For this review, take the finished solid that the model builds, in its own axes (mm). Give positions to 0.01 mm unless a question says otherwise; leave off trailing zeros. Write each loop counter-clockwise with the first axis right and the second up, starting at its lowest first coordinate (ties: lowest second). Pieces come first, ordered by that corner, then holes. Notation, with made-up numbers: M 15.25,-8 L 35.25,-8 A18 ccw 35.25,21 Z; hole C 65.25,74 d1. An arc over 180 degrees is marked long. One line per item, written item: value. Start each with the question number.
Item 1: Consider section B-B, the plane y = -89. Write out the cut boundary in (x, z), and give its area (3 significant figures).
Item 2: Consider section C-C, the plane z = 162. Write out the cut boundary in (x, y).
Item 3: Clearance check with flat-ended pins moving along their axes: pin 1 Ø5 at (x, y) = (88.5, -20) entering from -Z; pin 2 Ø2 at (x, z) = (100.5, 188.5) entering from -Y; pin 3 Ø8 at (x, z) = (53.5, 177) entering from +Y. State where each tip first meets the part, or that it passes through.
Item 4: Consider section A-A, the plane x = 68. Write out the cut boundary in (y, z), and give its area (3 significant figures).
Item 5: To check wall thickness, follow probe 1 along Y at (x, z) = (124.5, 189); probe 2 along Y at (x, z) = (128, 117.5); probe 3 along Z at (x, y) = (110.5, -106). State the ranges of each line that lie inside material, in increasing order.
```python
from build123d import *

# Parameters (mm, degrees)
BOSS_EXTRUDE1_DEPTH = 146.2024


with BuildPart() as part:
    # Sketch1 → Boss-Extrude1 (new body)
    with BuildSketch(Plane(origin=(0, 0, 0), x_dir=(0, 0, -1), z_dir=(1, 0, 0))):
        with BuildLine():
            Line((-213.527987278, -167.865893887), (-212.262670256, -168.824606088))
            ThreePointArc((-212.262670256, -168.824606088), (-116.43523539, -71.82151681), (1.233217804, -2.925713414))
            Line((1.233217804, -2.925713414), (0.616608902, -1.462856707))
            ThreePointArc((0.616608902, -1.462856707), (-117.409376916, -70.568039828), (-213.527987278, -167.865893887))
        make_face()
        with BuildLine():
            Line((-214.793304301, -166.907181687), (-213.527987278, -167.865893887))
            ThreePointArc((-213.527987278, -167.865893887), (-117.409376916, -70.568039828), (0.616608902, -1.462856707))
            Line((0.616608902, -1.462856707), (0, 0))
            ThreePointArc((0, 0), (-118.383518443, -69.314562846), (-214.793304301, -166.907181687))
        make_face()
    extrude(amount=BOSS_EXTRUDE1_DEPTH)


solid = part.part
```
Model answer:
1. outline: M 0,137.4 L 146.2,137.4 L 146.2,142.23 L 0,142.23 Z
1. area: 707 mm2
2. outline: M 0,-111.67 L 146.2,-111.67 L 146.2,-107.23 L 0,-107.23 Z
3. pin 1: stops at z = 30.37
3. pin 2: stops at y = -140.84
3. pin 3: stops at y = -118.23
4. outline: M -168.82,212.26 A522.33 cw -2.93,-1.23 L 0,0 A525.5 ccw -166.91,214.79 Z
4. area: 871 mm2
5. probe 1: y = -140.27 to -135.47
5. probe 2: y = -72.65 to -68.63
5. probe 3: z = 156.14 to 160.73
